Autodesk Inventor part; units mm, degrees
ref_plane "YZ Plane" through (0, 0, 0) normal (1, 0, 0) x (0, 1, 0)
ref_plane "XZ Plane" through (0, 0, 0) normal (0, 1, 0) x (-1, 0, 0)
ref_plane "XY Plane" through (0, 0, 0) normal (0, 0, 1) x (1, 0, 0)
sketch "Sketch1" plane through (0, 0, 0) normal (0, 1, 0) x (-1, 0, 0)
  line L0 (-25.25, 42.75) -> (25.25, 42.75)
  line L1 (28.25, 39.75) -> (28.25, -40.75)
  line L2 (26.25, -42.75) -> (-25.25, -42.75)
  line L3 (-28.25, -39.75) -> (-28.25, 39.75)
  line L4 (-28.25, 42.75) -> (28.25, -42.75) construction
  line L5 (28.25, 42.75) -> (-28.25, -42.75) construction
  arc A0 (26.25, -42.75) -> (28.25, -40.75) centre (26.25, -40.75) ccw
  arc A1 (-28.25, -39.75) -> (-25.25, -42.75) centre (-25.25, -39.75) ccw
  arc A2 (-25.25, 42.75) -> (-28.25, 39.75) centre (-25.25, 39.75) ccw
  arc A3 (28.25, 39.75) -> (25.25, 42.75) centre (25.25, 39.75) ccw
  line L6 (30.25, -40.75) -> (30.25, 39.75)
  arc A4 (30.25, 39.75) -> (25.25, 44.75) centre (25.25, 39.75) ccw
  line L7 (25.25, 44.75) -> (-25.25, 44.75)
  arc A5 (-25.25, 44.75) -> (-30.25, 39.75) centre (-25.25, 39.75) ccw
  line L8 (-30.25, 39.75) -> (-30.25, -39.75)
  arc A6 (-30.25, -39.75) -> (-25.25, -44.75) centre (-25.25, -39.75) ccw
  line L9 (-25.25, -44.75) -> (26.25, -44.75)
  arc A7 (26.25, -44.75) -> (30.25, -40.75) centre (26.25, -40.75) ccw
  point P0 (0, 0)
  dimension "d0" = 56.5
  dimension "d1" = 85.5
  dimension "d2" = 2
  dimension "d3" = 3
  dimension "d4" = 2
extrude "Extrusion1" add sketch "Sketch1" along normal blind 3
sketch "Sketch2" plane through (0, 0, 0) normal (0, -1, 0) x (1, 0, 0)
  arc A0 (-25.25, 44.75) -> (-30.25, 39.75) centre (-25.25, 39.75) ccw
  line L0 (-25.25, 44.75) -> (25.25, 44.75)
  arc A1 (30.25, 39.75) -> (25.25, 44.75) centre (25.25, 39.75) ccw
  line L1 (30.25, 39.75) -> (30.25, -39.75)
  arc A2 (25.25, -44.75) -> (30.25, -39.75) centre (25.25, -39.75) ccw
  line L2 (25.25, -44.75) -> (-26.25, -44.75)
  arc A3 (-30.25, -40.75) -> (-26.25, -44.75) centre (-26.25, -40.75) ccw
  line L3 (-30.25, -40.75) -> (-30.25, 39.75)
  line L4 (-26.25, -44.75) -> (25.25, -44.75)
  line L5 (30.25, -39.75) -> (30.25, 39.75)
  line L6 (25.25, 44.75) -> (-25.25, 44.75)
  line L7 (-30.25, 39.75) -> (-30.25, -40.75)
  line L8 (-30, -44.5) -> (30, 44.5) construction
  line L9 (30, -44.5) -> (-30, 44.5) construction
  arc A4 (-25.25, 44.75) -> (-30.25, 39.75) centre (-25.25, 39.75) ccw
  arc A5 (30.25, 39.75) -> (25.25, 44.75) centre (25.25, 39.75) ccw
  arc A6 (25.25, -42.75) -> (28.25, -39.75) centre (25.25, -39.75) ccw
  arc A7 (25.25, -44.75) -> (30.25, -39.75) centre (25.25, -39.75) ccw
  arc A8 (-30.25, -40.75) -> (-26.25, -44.75) centre (-26.25, -40.75) ccw
  line L10 (25.25, 40.75) -> (-25.25, 40.75)
  arc A9 (-25.25, 40.75) -> (-26.25, 39.75) centre (-25.25, 39.75) ccw
  line L11 (-26.25, 39.75) -> (-26.25, -40.75)
  line L12 (-26.25, -40.75) -> (25.25, -40.75)
  arc A10 (25.25, -40.75) -> (26.25, -39.75) centre (25.25, -39.75) ccw
  line L13 (26.25, -39.75) -> (26.25, 39.75)
  arc A11 (26.25, 39.75) -> (25.25, 40.75) centre (25.25, 39.75) ccw
  point P0 (0, 0)
  point P1 (-26.25, -40.75)
  dimension "d12" = 4
extrude "Extrusion2" add sketch "Sketch2" along normal blind 2.5
sketch "Sketch3" plane through (25.25, 3, -44.75) normal (0, 0, -1) x (-1, 0, 0)
  line L0 (51.5, -5.5) -> (51.5, 0)
  line L1 (51.5, 0) -> (0, 0)
  line L2 (0, 0) -> (0, 1.5)
  line L3 (0, 1.5) -> (51.5, 1.5)
  line L4 (51.5, 1.5) -> (51.5, 0)
  point P0 (25.25, -3)
  dimension "d9" = 1.5
extrude "Extrusion3" add sketch "Sketch3" against normal blind 2
sketch "Sketch4" plane through (0, -2.5, 0) normal (0, -1, 0) x (1, 0, 0)
  line L0 (25.25, 44.75) -> (-25.25, 44.75)
  line L1 (-30.25, 39.75) -> (-30.25, -40.75)
  line L2 (-26.25, -44.75) -> (25.25, -44.75)
  line L3 (30.25, -39.75) -> (30.25, 39.75)
  line L4 (30, 44.5) -> (-30, -44.5) construction
  line L5 (-30, 44.5) -> (30, -44.5) construction
  line L6 (-26.25, -44.75) -> (25.25, -44.75)
  line L7 (-30.25, 39.75) -> (-30.25, -40.75)
  arc A0 (25.25, -44.75) -> (30.25, -39.75) centre (25.25, -39.75) ccw
  arc A1 (-30.25, -40.75) -> (-26.25, -44.75) centre (-26.25, -40.75) ccw
  arc A2 (-25.25, 44.75) -> (-30.25, 39.75) centre (-25.25, 39.75) ccw
  arc A3 (30.25, 39.75) -> (25.25, 44.75) centre (25.25, 39.75) ccw
  arc A4 (25.25, -44.75) -> (30.25, -39.75) centre (25.25, -39.75) ccw
  line L8 (25.25, -40.75) -> (-26.25, -40.75)
  arc A5 (-30.25, -40.75) -> (-26.25, -44.75) centre (-26.25, -40.75) ccw
  arc A6 (-25.25, 44.75) -> (-30.25, 39.75) centre (-25.25, 39.75) ccw
  arc A7 (30.25, 39.75) -> (25.25, 44.75) centre (25.25, 39.75) ccw
  line L9 (25.25, 44.75) -> (-25.25, 44.75)
  point P0 (0, 0)
  point P1 (-30.25, 39.75)
  point P2 (-30.25, -40.75)
  point P3 (25.25, -44.75)
extrude "Extrusion4" add sketch "Sketch4" along normal blind 2.5
sketch "Sketch5" plane through (25.25, 4.5, -44.75) normal (0, 0, -1) x (-1, 0, 0)
  line L0 (51.5, -9.5) -> (0, -9.5)
  line L1 (18.25, -9.5) -> (32.25, -9.5)
  line L2 (32.25, -9.5) -> (32.25, -3.5)
  line L3 (32.25, -3.5) -> (18.25, -3.5)
  line L4 (18.25, -3.5) -> (18.25, -9.5)
  line L5 (18.25, -9.5) -> (32.25, -3.5) construction
  line L6 (32.25, -9.5) -> (18.25, -3.5) construction
  point P0 (25.25, -4.5)
  point P1 (25.25, -6.5)
  dimension "d16" = 14
  dimension "d17" = 0
  dimension "d18" = 6
extrude "Extrusion5" cut sketch "Sketch5" against normal blind 10
sketch "Sketch6" plane through (-30.25, 3, -40.75) normal (-1, 0, 0) x (0, 0, 1)
  line L0 (1, 0) -> (80.5, 0)
  line L1 (4.6696, 0) -> (13.8622, 0)
  line L2 (13.8622, 0) -> (13.8622, -2)
  line L3 (13.8622, -2) -> (4.6696, -2)
  line L4 (4.6696, -2) -> (4.6696, 0)
  line L5 (20.7687, 0) -> (27.5371, 0)
  line L6 (27.5371, 0) -> (27.5371, -2)
  line L7 (27.5371, -2) -> (20.7687, -2)
  line L8 (20.7687, -2) -> (20.7687, 0)
  line L9 (34.3481, 0) -> (41.1165, 0)
  line L10 (41.1165, 0) -> (41.1165, -2)
  line L11 (41.1165, -2) -> (34.3481, -2)
  line L12 (34.3481, -2) -> (34.3481, 0)
  arc A0 (49.8136, 0) -> (55.8136, 0) centre (52.8136, 1.25) ccw
  line L13 (-2, 1.5) -> (-2, 0)
  line L14 (80.5, -8) -> (0, -8)
  line L15 (49.8136, 0) -> (55.8136, 0)
  point P0 (40.75, -3)
  dimension "d21" = 6.6696
  dimension "d22" = 9.1926
  dimension "d23" = 22.7687
  dimension "d25" = 6.7684
  dimension "d26" = 6.7684
  dimension "d27" = 36.3481
  dimension "d28" = 51.8136
  dimension "d29" = 6
  dimension "d30" = 2
extrude "Extrusion6" cut sketch "Sketch6" against normal up to surface (2 mm away)
sketch "Sketch7" plane through (-25.25, 3, 44.75) normal (0, 0, 1) x (1, 0, 0)
  line L0 (50.5, 0) -> (0, 0)
  line L1 (-0.7188, 0) -> (12.8798, 0)
  line L2 (12.8798, 0) -> (12.8798, -2)
  line L3 (12.8798, -2) -> (-0.7188, -2)
  line L4 (-0.7188, -2) -> (-0.7188, 0)
  line L5 (17.4418, 0) -> (31.0404, 0)
  line L6 (31.0404, 0) -> (31.0404, -2)
  line L7 (31.0404, -2) -> (17.4418, -2)
  line L8 (17.4418, -2) -> (17.4418, 0)
  line L9 (34.977, 0) -> (51.34, 0)
  line L10 (51.34, 0) -> (51.34, -2)
  line L11 (51.34, -2) -> (34.977, -2)
  line L12 (34.977, -2) -> (34.977, 0)
  line L13 (-3, -3) -> (-3, 0)
  point P0 (25.25, -3)
  dimension "d33" = 2
  dimension "d34" = 2.2812
  dimension "d35" = 13.5986
  dimension "d36" = 20.4418
  dimension "d37" = 13.5986
  dimension "d38" = 37.977
  dimension "d39" = 16.363
extrude "Extrusion7" cut sketch "Sketch7" against normal blind 5
properties part number "piholder-proto-v5"
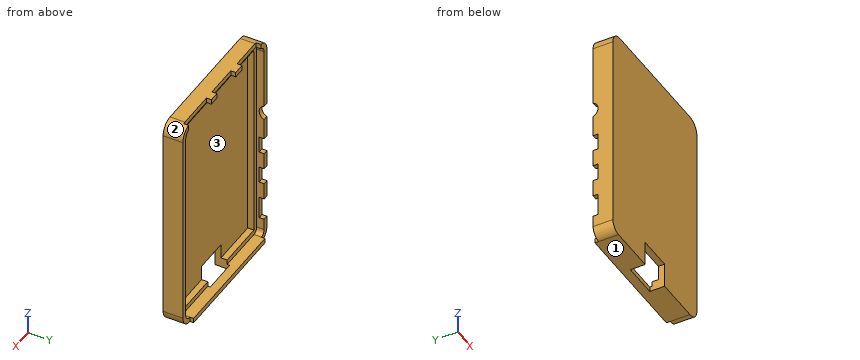
Verification items for the finished model (mm, model axes). Face numbers are marked on the shaded views. Give positions to 0.01 mm unless a question says otherwise; leave off trailing zeros. Loops run counter-clockwise (first coordinate to the right, second up) from the corner with the lowest first, then second, coordinate; pieces in that order, holes last. Notation, with made-up numbers: (-4, 57.25) - (39, 57.25) arc R16 cw to (39, 76.25) - close; hole circle Ø6 at (-6.75, -14.5). An arc over 180 degrees is marked (long way). Write item = value, one per line. Start each with the question number.
Q1. Depth check by flat-ended pin: P1, Ø0.8, axis at x = -3, y = -1, coming from the -Z side; P2, Ø2, axis at x = -10, z = 43.5, coming from the +Y side; P3, Ø0.6, axis at x = 0, z = -44, coming from the -Y side. Enter the tip coordinate at first touch or a pass-through.
Q2. Cross-section at A-A, the plane x = 1.5. Enter the section's corners in (y, z), and give its area (3 significant figures).
Q3. Thickness scan on line 1 (Z direction, x = 12.5, y = -1.25); line 2 (X direction, y = -0.5, z = 25); line 3 (X direction, y = 2, z = 23.5). Record the ranges inside material, lowest first.
Q4. Cross-section at B-B, the plane z = -29.5. Enter the section's corners in (x, y), and give its area (3 significant figures).
Q5. Mould release check, pull along Z, two halves, no side actions. Record for the marked faces 1, 2 and 3: released by +Z, released by -Z, zero draft, split by the parting line, or undercut.
Q6. Cross-section at C-C, the plane y = -4. Enter the section's corners in (x, z), and give its area (3 significant figures).
Answer key:
q1.P1 = 40.75
q1.P2 = 3
q1.P3 = 1
q2.outline = (-5, -34.75) - (-2.5, -34.75) - (-2.5, 40.75) - (0, 40.75) - (0, 42.75) - (1, 42.75) - (1, 44.75) - (-5, 44.75) - close; (1, -44.75) - (4.5, -44.75) - (4.5, -42.75) - (1, -42.75) - close
q2.area = 218 mm^2
q3.line_1 = -44.75 to -40.75, 40.75 to 44.75
q3.line_2 = -30.25 to -26.25, 26.25 to 30.25
q3.line_3 = -30.25 to -28.25, 28.25 to 30.25
q4.outline = (-30.25, -5) - (30.25, -5) - (30.25, 3) - (28.25, 3) - (28.25, 0) - (26.25, 0) - (26.25, -2.5) - (-26.25, -2.5) - (-26.25, 0) - (-28.25, 0) - (-28.25, 1) - (-30.25, 1) - close
q4.area = 179 mm^2
q5.face_1 = released by -Z
q5.face_2 = released by +Z
q5.face_3 = undercut
q6.outline = (-30.25, -40.75) arc R4 ccw to (-26.25, -44.75) - (-7, -44.75) - (-7, -34.75) - (7, -34.75) - (7, -44.75) - (25.25, -44.75) arc R5 ccw to (30.25, -39.75) - (30.25, 39.75) arc R5 ccw to (25.25, 44.75) - (-25.25, 44.75) arc R5 ccw to (-30.25, 39.75) - close
q6.area = 5,260 mm^2
